Build history of the part. All positions in model axes, mm. A direction names the side the tool comes from. Round coordinates to 2 decimals unless told otherwise and drop trailing zeros. Write each loop counter-clockwise with the first axis right and the second up, starting at its lowest first coordinate (ties: lowest second). Pieces come first, ordered by that corner, then holes. Notation, with made-up numbers: (-9.75, 69.25) -> (43.25, 69.25) arc R23 cw to (43.25, 95.25) -> close; hole circle Ø6 at (-28.75, 66.25). An arc over 180 degrees is marked (long way). Answer in a Markdown table with one row per item.
```python
from build123d import *

# Parameters (mm, degrees)
F1_DEPTH = 6.5
F2_DEPTH = 1.9


with BuildPart() as f1:
    # F0 (on Top) → F1 (new body)
    with BuildSketch(Plane.XY):
        with BuildLine():
            Line((-8.899431151, 5.8993360586), (-10.899431151, 5.8993360586))
            ThreePointArc((-10.899431151, 5.8993360586), (-11.4896109869, 4.4745158946), (-12.914431151, 3.8843360586))
            Line((-12.914431151, 3.8843360586), (-12.914431151, 1.8843360586))
            ThreePointArc((-12.914431151, 1.8843360586), (-10.0753974245, 3.0603023322), (-8.899431151, 5.8993360586))
        make_face()
        with BuildLine():
            ThreePointArc((-12.914431151, 3.8843360586), (-14.3392513151, 7.3241562227), (-10.899431151, 5.8993360586))
            Line((-10.899431151, 5.8993360586), (-8.899431151, 5.8993360586))
            ThreePointArc((-8.899431151, 5.8993360586), (-10.0753974245, 8.7383697851), (-12.914431151, 9.9143360586))
            ThreePointArc((-12.914431151, 9.9143360586), (-15.7534648775, 8.7383697851), (-16.929431151, 5.8993360586))
            ThreePointArc((-16.929431151, 5.8993360586), (-15.7534648775, 3.0603023322), (-12.914431151, 1.8843360586))
            Line((-12.914431151, 1.8843360586), (-12.914431151, 3.8843360586))
        make_face()
    extrude(amount=F1_DEPTH)



with BuildPart() as f1b:
    # F0 (on Top) → F1, piece 2 (new body)
    with BuildSketch(Plane.XY):
        with BuildLine():
            ThreePointArc((17.085568849, 9.9143360586), (14.2465351225, 8.7383697851), (13.070568849, 5.8993360586))
            Line((13.070568849, 5.8993360586), (15.070568849, 5.8993360586))
            ThreePointArc((15.070568849, 5.8993360586), (17.085568849, 7.9143360586), (19.100568849, 5.8993360586))
            ThreePointArc((19.100568849, 5.8993360586), (18.5103890131, 4.4745158946), (17.085568849, 3.8843360586))
            Line((17.085568849, 3.8843360586), (17.085568849, 1.8843360586))
            ThreePointArc((17.085568849, 1.8843360586), (19.9246025755, 3.0603023322), (21.100568849, 5.8993360586))
            ThreePointArc((21.100568849, 5.8993360586), (19.9246025755, 8.7383697851), (17.085568849, 9.9143360586))
        make_face()
        with BuildLine():
            Line((15.070568849, 5.8993360586), (13.070568849, 5.8993360586))
            ThreePointArc((13.070568849, 5.8993360586), (14.2465351225, 3.0603023322), (17.085568849, 1.8843360586))
            Line((17.085568849, 1.8843360586), (17.085568849, 3.8843360586))
            ThreePointArc((17.085568849, 3.8843360586), (15.6607486849, 4.4745158946), (15.070568849, 5.8993360586))
        make_face()
    extrude(amount=F1_DEPTH)


with BuildPart() as f1c:
    # F0 (on Top) → F1, piece 3 (new body)
    with BuildSketch(Plane.XY):
        with BuildLine():
            ThreePointArc((21.100568849, -24.1006639414), (19.9246025755, -21.2616302149), (17.085568849, -20.0856639414))
            Line((17.085568849, -20.0856639414), (17.085568849, -22.0856639414))
            ThreePointArc((17.085568849, -22.0856639414), (18.5103890131, -22.6758437773), (19.100568849, -24.1006639414))
            ThreePointArc((19.100568849, -24.1006639414), (17.085568849, -26.1156639414), (15.070568849, -24.1006639414))
            Line((15.070568849, -24.1006639414), (13.070568849, -24.1006639414))
            ThreePointArc((13.070568849, -24.1006639414), (14.2465351225, -26.9396976678), (17.085568849, -28.1156639414))
            ThreePointArc((17.085568849, -28.1156639414), (19.9246025755, -26.9396976678), (21.100568849, -24.1006639414))
        make_face()
        with BuildLine():
            Line((17.085568849, -22.0856639414), (17.085568849, -20.0856639414))
            ThreePointArc((17.085568849, -20.0856639414), (14.2465351225, -21.2616302149), (13.070568849, -24.1006639414))
            Line((13.070568849, -24.1006639414), (15.070568849, -24.1006639414))
            ThreePointArc((15.070568849, -24.1006639414), (15.6607486849, -22.6758437773), (17.085568849, -22.0856639414))
        make_face()
    extrude(amount=F1_DEPTH)


with BuildPart() as f1d:
    # F0 (on Top) → F1, piece 4 (new body)
    with BuildSketch(Plane.XY):
        with BuildLine():
            Line((-12.914431151, -22.0856639414), (-12.914431151, -20.0856639414))
            ThreePointArc((-12.914431151, -20.0856639414), (-15.7534648775, -21.2616302149), (-16.929431151, -24.1006639414))
            ThreePointArc((-16.929431151, -24.1006639414), (-15.7534648775, -26.9396976678), (-12.914431151, -28.1156639414))
            ThreePointArc((-12.914431151, -28.1156639414), (-10.0753974245, -26.9396976678), (-8.899431151, -24.1006639414))
            Line((-8.899431151, -24.1006639414), (-10.899431151, -24.1006639414))
            ThreePointArc((-10.899431151, -24.1006639414), (-14.3392513151, -25.5254841054), (-12.914431151, -22.0856639414))
        make_face()
        with BuildLine():
            ThreePointArc((-8.899431151, -24.1006639414), (-10.0753974245, -21.2616302149), (-12.914431151, -20.0856639414))
            Line((-12.914431151, -20.0856639414), (-12.914431151, -22.0856639414))
            ThreePointArc((-12.914431151, -22.0856639414), (-11.4896109869, -22.6758437773), (-10.899431151, -24.1006639414))
            Line((-10.899431151, -24.1006639414), (-8.899431151, -24.1006639414))
        make_face()
    extrude(amount=F1_DEPTH)


with BuildPart() as f1_1:
    add(f1.part)

    add(f1b.part)  # F2 merges F1b

    add(f1c.part)  # F2 merges F1c

    add(f1d.part)  # F2 merges F1d
    # F0 (on Top) → F2 (join)
    with BuildSketch(Plane.XY):
        with BuildLine():
            ThreePointArc((-12.914431151, 3.8843360586), (-14.3392513151, 7.3241562227), (-10.899431151, 5.8993360586))
            Line((-10.899431151, 5.8993360586), (-8.899431151, 5.8993360586))
            ThreePointArc((-8.899431151, 5.8993360586), (-10.0753974245, 8.7383697851), (-12.914431151, 9.9143360586))
            ThreePointArc((-12.914431151, 9.9143360586), (-15.7534648775, 8.7383697851), (-16.929431151, 5.8993360586))
            ThreePointArc((-16.929431151, 5.8993360586), (-15.7534648775, 3.0603023322), (-12.914431151, 1.8843360586))
            Line((-12.914431151, 1.8843360586), (-12.914431151, 3.8843360586))
        make_face()
        with BuildLine():
            ThreePointArc((-12.914431151, 9.9143360586), (-10.0753974245, 8.7383697851), (-8.899431151, 5.8993360586))
            Line((-8.899431151, 5.8993360586), (13.070568849, 5.8993360586))
            ThreePointArc((13.070568849, 5.8993360586), (14.2465351225, 8.7383697851), (17.085568849, 9.9143360586))
            Line((17.085568849, 9.9143360586), (-12.914431151, 9.9143360586))
        make_face()
        with BuildLine():
            Line((-12.914431151, -20.0856639414), (-12.914431151, 1.8843360586))
            ThreePointArc((-12.914431151, 1.8843360586), (-15.7534648775, 3.0603023322), (-16.929431151, 5.8993360586))
            Line((-16.929431151, 5.8993360586), (-16.929431151, -24.1006639414))
            ThreePointArc((-16.929431151, -24.1006639414), (-15.7534648775, -21.2616302149), (-12.914431151, -20.0856639414))
        make_face()
        with BuildLine():
            ThreePointArc((17.085568849, 9.9143360586), (14.2465351225, 8.7383697851), (13.070568849, 5.8993360586))
            Line((13.070568849, 5.8993360586), (15.070568849, 5.8993360586))
            ThreePointArc((15.070568849, 5.8993360586), (17.085568849, 7.9143360586), (19.100568849, 5.8993360586))
            ThreePointArc((19.100568849, 5.8993360586), (18.5103890131, 4.4745158946), (17.085568849, 3.8843360586))
            Line((17.085568849, 3.8843360586), (17.085568849, 1.8843360586))
            ThreePointArc((17.085568849, 1.8843360586), (19.9246025755, 3.0603023322), (21.100568849, 5.8993360586))
            ThreePointArc((21.100568849, 5.8993360586), (19.9246025755, 8.7383697851), (17.085568849, 9.9143360586))
        make_face()
        with BuildLine():
            Line((-12.914431151, -22.0856639414), (-12.914431151, -20.0856639414))
            ThreePointArc((-12.914431151, -20.0856639414), (-15.7534648775, -21.2616302149), (-16.929431151, -24.1006639414))
            ThreePointArc((-16.929431151, -24.1006639414), (-15.7534648775, -26.9396976678), (-12.914431151, -28.1156639414))
            ThreePointArc((-12.914431151, -28.1156639414), (-10.0753974245, -26.9396976678), (-8.899431151, -24.1006639414))
            Line((-8.899431151, -24.1006639414), (-10.899431151, -24.1006639414))
            ThreePointArc((-10.899431151, -24.1006639414), (-14.3392513151, -25.5254841054), (-12.914431151, -22.0856639414))
        make_face()
        with BuildLine():
            ThreePointArc((21.100568849, 5.8993360586), (19.9246025755, 3.0603023322), (17.085568849, 1.8843360586))
            Line((17.085568849, 1.8843360586), (17.085568849, -20.0856639414))
            ThreePointArc((17.085568849, -20.0856639414), (19.9246025755, -21.2616302149), (21.100568849, -24.1006639414))
            Line((21.100568849, -24.1006639414), (21.100568849, 5.8993360586))
        make_face()
        with BuildLine():
            Line((13.070568849, -24.1006639414), (-8.899431151, -24.1006639414))
            ThreePointArc((-8.899431151, -24.1006639414), (-10.0753974245, -26.9396976678), (-12.914431151, -28.1156639414))
            Line((-12.914431151, -28.1156639414), (17.085568849, -28.1156639414))
            ThreePointArc((17.085568849, -28.1156639414), (14.2465351225, -26.9396976678), (13.070568849, -24.1006639414))
        make_face()
        with BuildLine():
            ThreePointArc((21.100568849, -24.1006639414), (19.9246025755, -21.2616302149), (17.085568849, -20.0856639414))
            Line((17.085568849, -20.0856639414), (17.085568849, -22.0856639414))
            ThreePointArc((17.085568849, -22.0856639414), (18.5103890131, -22.6758437773), (19.100568849, -24.1006639414))
            ThreePointArc((19.100568849, -24.1006639414), (17.085568849, -26.1156639414), (15.070568849, -24.1006639414))
            Line((15.070568849, -24.1006639414), (13.070568849, -24.1006639414))
            ThreePointArc((13.070568849, -24.1006639414), (14.2465351225, -26.9396976678), (17.085568849, -28.1156639414))
            ThreePointArc((17.085568849, -28.1156639414), (19.9246025755, -26.9396976678), (21.100568849, -24.1006639414))
        make_face()
        with BuildLine():
            Line((2.085568849, -5.0856639414), (-8.899431151, 5.8993360586))
            ThreePointArc((-8.899431151, 5.8993360586), (-10.0753974245, 3.0603023322), (-12.914431151, 1.8843360586))
            Line((-12.914431151, 1.8843360586), (-1.929431151, -9.1006639414))
            Line((-1.929431151, -9.1006639414), (2.085568849, -5.0856639414))
        make_face()
        with BuildLine():
            ThreePointArc((17.085568849, 1.8843360586), (14.2465351225, 3.0603023322), (13.070568849, 5.8993360586))
            Line((13.070568849, 5.8993360586), (2.085568849, -5.0856639414))
            Line((2.085568849, -5.0856639414), (6.100568849, -9.1006639414))
            Line((6.100568849, -9.1006639414), (17.085568849, 1.8843360586))
        make_face()
        Polygon((6.100568849, -9.1006639414), (2.085568849, -5.0856639414), (-1.929431151, -9.1006639414), (2.085568849, -13.1156639414), align=None)
        with BuildLine():
            Line((17.085568849, -20.0856639414), (6.100568849, -9.1006639414))
            Line((6.100568849, -9.1006639414), (2.085568849, -13.1156639414))
            Line((2.085568849, -13.1156639414), (13.070568849, -24.1006639414))
            ThreePointArc((13.070568849, -24.1006639414), (14.2465351225, -21.2616302149), (17.085568849, -20.0856639414))
        make_face()
        with BuildLine():
            Line((-1.929431151, -9.1006639414), (-12.914431151, -20.0856639414))
            ThreePointArc((-12.914431151, -20.0856639414), (-10.0753974245, -21.2616302149), (-8.899431151, -24.1006639414))
            Line((-8.899431151, -24.1006639414), (2.085568849, -13.1156639414))
            Line((2.085568849, -13.1156639414), (-1.929431151, -9.1006639414))
        make_face()
    extrude(amount=F2_DEPTH)


solid = f1_1.part
```
Q1. Saw through at C-C on y = -25. Write the cut outline in (x, z).
A:
| item | result |
|---|---|
| outline | (-16.83, 0) -> (-14.72, 0) -> (-14.72, 6.5) -> (-16.83, 6.5) -> close; (-11.11, 0) -> (15.28, 0) -> (15.28, 6.5) -> (13.17, 6.5) -> (13.17, 1.9) -> (-9, 1.9) -> (-9, 6.5) -> (-11.11, 6.5) -> close; (18.89, 0) -> (21, 0) -> (21, 6.5) -> (18.89, 6.5) -> close |
Q2. Saw through at A-A on z = 3.5. Write the cut outline in (x, y) (3 decimals), plus the area to 3 significant figures.
A:
| item | result |
|---|---|
| outline | circle Ø8.03 at (-12.914, -24.101); circle Ø8.03 at (-12.914, 5.899); circle Ø8.03 at (17.086, -24.101); circle Ø8.03 at (17.086, 5.899); hole circle Ø4.03 at (-12.914, -24.101); hole circle Ø4.03 at (-12.914, 5.899); hole circle Ø4.03 at (17.086, -24.101); hole circle Ø4.03 at (17.086, 5.899) |
| area | 152 mm² |
Q3. Saw through at B-B on x = 14.5. Write the cut outline in (y, z).
A:
| item | result |
|---|---|
| outline | (-28.12, 0) -> (-17.5, 0) -> (-17.5, 1.9) -> (-21.03, 1.9) -> (-21.03, 6.5) -> (-27.17, 6.5) -> (-27.17, 1.9) -> (-28.12, 1.9) -> close; (-0.7, 0) -> (9.91, 0) -> (9.91, 1.9) -> (8.97, 1.9) -> (8.97, 6.5) -> (2.83, 6.5) -> (2.83, 1.9) -> (-0.7, 1.9) -> close |
Q4. Wall check: line 1 (Y direction, x = 17, z = 4); line 2 (Y direction, x = 7, z = 1.5); line 3 (Y direction, x = 19.5, z = 6.25). Give the ranges that are in metal, low to high. Write a range as [from, to].
A:
| item | result |
|---|---|
| line 1 | [-28.11, -26.11], [-22.09, -20.09], [1.89, 3.89], [7.91, 9.91] |
| line 2 | [-28.12, -24.1], [-18.03, -10], [-8.2, -0.17], [5.9, 9.91] |
| line 3 | [-27.31, -20.89], [2.69, 9.11] |
Q5. Drop flat-ended pins along their axis: P1, Ø1.2, axis at x = -2.5, y = -26.5, coming from the +Z side; P2, Ø2, axis at y = -20.5, z = 5, coming from the -X side; P3, Ø1, axis at x = -2.5, y = 4.5, coming from the -Z side. Give the stop position or say it passes through.
A:
| item | result |
|---|---|
| P1 | z = 1.9 |
| P2 | x = -15.97 |
| P3 | through |
Q6. Two-plate mould, pull along Y, no slides. Class faces 1 (the flat face through (2, -28.116, 1)), 2 (the flat face through (-7.5, -3.53, 0.94)), 3 (the flat face through (2, -26, 1.9)), 4 (the flat face through (2, 9.914, 1)): released by +Y, released by -Y, zero draft, split by the parting line, or undercut.
A:
| item | result |
|---|---|
| face 1 | released by -Y |
| face 2 | undercut |
| face 3 | zero draft |
| face 4 | released by +Y |
Q7. Which spindle directions (+Z, -Z, +X, -X, +Y, -Y) get a long thin tool onto all of the face, cutting with end or side? Do faces 5 (the flat face through (15, -25, 6.5)), 6 (the flat face through (17.086, -9, 1)). Say none if no direction does.
A:
| item | result |
|---|---|
| face 5 | +Z, +X, -X, +Y, -Y |
| face 6 | +Z, -Z |
Q8. Saw through at D-D on x = 3. Write the cut outline in (y, z).
A:
| item | result |
|---|---|
| outline | (-28.12, 0) -> (-24.1, 0) -> (-24.1, 1.9) -> (-28.12, 1.9) -> close; (-14.03, 0) -> (-4.17, 0) -> (-4.17, 1.9) -> (-14.03, 1.9) -> close; (5.9, 0) -> (9.91, 0) -> (9.91, 1.9) -> (5.9, 1.9) -> close |
